Read the model definition and answer for the solid it produces. Units are mm, in the model's axes. Round coordinates to 2 decimals unless told otherwise and drop trailing zeros. Order: outer loops, then holes, each group sorted by start corner. A loop starts at its lowest first (then second) coordinate and runs counter-clockwise, first axis right, second up. Notation, with made-up numbers: (-13.5, 56) -> (7.5, 56) arc R34 ccw to (7.5, 87) -> close; hole circle Ø4 at (58, 41). An arc over 180 degrees is marked (long way). Use a Markdown table: item, result. Add a question column.
1. Section B-B, the plane z = -256 is taken. Give the vertices of the cut face in (x, y).
2. Consider L1, parallel to Z at x = 10.25, y = 0; L2, parallel to X at y = -0.55, z = -577; L3, parallel to X at y = 0, z = -534. Determine where each line is inside the solid, lowest interval first. Write a range as [from, to].
3. Given pin 1 (2 mm diameter, centred on x = 16.5, y = 2, fed in from -Z), flat-ended and moving along its own axis, determine where the tip first touches the part or whether it passes through.
4. Section A-A, the plane y = 0 is taken. Give the vertices of the cut face in (x, z) (1 decimal), then the cut area to 3 significant figures.
```python
from build123d import *

# Parameters (mm, degrees)
SKETCH2_R   = 2.38125
SKETCH2_R_2 = 1.82245


with BuildPart() as part:
    # Sweep1: sweep along a path in Sketch1
    with BuildLine(Plane(origin=(0, 0, 0), x_dir=(1, 0, 0), z_dir=(0, 1, 0))) as sweep1_path:
        Line((49.521745, 815.975), (49.521745, 34.925))
        ThreePointArc((49.521745, 34.925), (39.292449333, 10.229295667), (14.596745, 0))
        Line((14.596745, 0), (0, 0))
    # Sketch2 → Sweep1 (sweep)
    with BuildSketch(Plane(origin=(0, 0, 0), x_dir=(0, 0, -1), z_dir=(1, 0, 0))):
        Circle(SKETCH2_R)
        Circle(SKETCH2_R_2, mode=Mode.SUBTRACT)
    sweep(path=sweep1_path.line)


solid = part.part
```
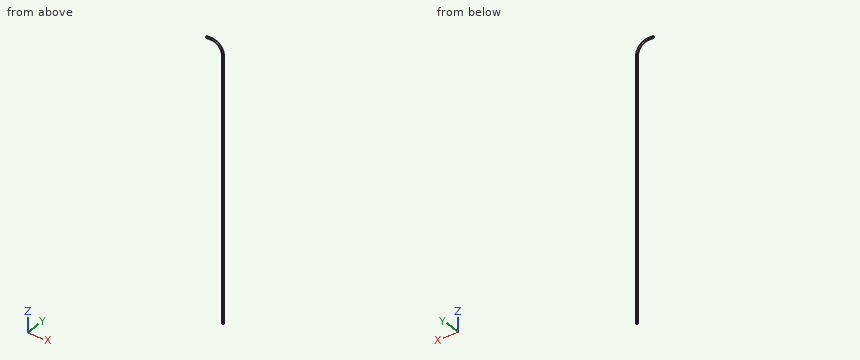
Verdict:
| question | item | result |
|---|---|---|
| 1 | outline | circle Ø4.76 at (49.52, 0); hole circle Ø3.64 at (49.52, 0) |
| 2 | L1 | z = [-2.38, -1.82], [1.82, 2.38] |
| 2 | L2 | x = [47.2, 47.78], [51.26, 51.84] |
| 2 | L3 | x = [47.14, 47.7], [51.34, 51.9] |
| 3 | pin 1 | stops at z = -2.22 |
| 4 | outline | (0, -2.4) -> (14.6, -2.4) arc R32.5 cw to (47.1, -34.9) -> (47.1, -816) -> (47.7, -816) -> (47.7, -34.9) arc R33.1 ccw to (14.6, -1.8) -> (0, -1.8) -> close; (0, 1.8) -> (14.6, 1.8) arc R36.7 cw to (51.3, -34.9) -> (51.3, -816) -> (51.9, -816) -> (51.9, -34.9) arc R37.3 ccw to (14.6, 2.4) -> (0, 2.4) -> close |
| 4 | area | 951 mm2 |
